The model under review builds one solid part; all positions refer to its coordinate system, in mm. Coordinates: 2 decimals unless noted, no trailing zeros. Write each loop counter-clockwise with the first axis right and the second up, starting at its lowest first coordinate (ties: lowest second). Pieces come first, ordered by that corner, then holes.
```python
from build123d import *

# Parameters (mm, degrees)
SKETCH1_W           = 50
SKETCH1_H           = 14
BOSS_EXTRUDE1_DEPTH = 2.2
SKETCH2_R           = 2.5
CUT_EXTRUDE1_DEPTH  = 27.054558142
FILLET1_R           = 0.1
FILLET2_R           = 0.1


with BuildPart() as part:
    # Sketch1 → Boss-Extrude1 (new body)
    with BuildSketch(Plane(origin=(0, 0, 0), x_dir=(0, 0, -1), z_dir=(1, 0, 0))):
        Rectangle(SKETCH1_W, SKETCH1_H)
    extrude(amount=BOSS_EXTRUDE1_DEPTH)

    # Sketch2 → Cut-Extrude1 (cut, through all)
    with BuildSketch(Plane(origin=(2.2, 0, 0), x_dir=(0, 0, -1), z_dir=(1, 0, 0))):
        with Locations((-20, 0)):
            Circle(SKETCH2_R)
    extrude(amount=-CUT_EXTRUDE1_DEPTH, mode=Mode.SUBTRACT)

    # Fillet1
    fillet1_edges = [part.edges().sort_by_distance(p)[0] for p in [
        (2.2, 0, -25),
    ]]
    fillet(fillet1_edges, radius=FILLET1_R)

    # Fillet2
    fillet2_edges = [part.edges().sort_by_distance(p)[0] for p in [
        (0, 0, -25),
    ]]
    fillet(fillet2_edges, radius=FILLET2_R)


solid = part.part
```
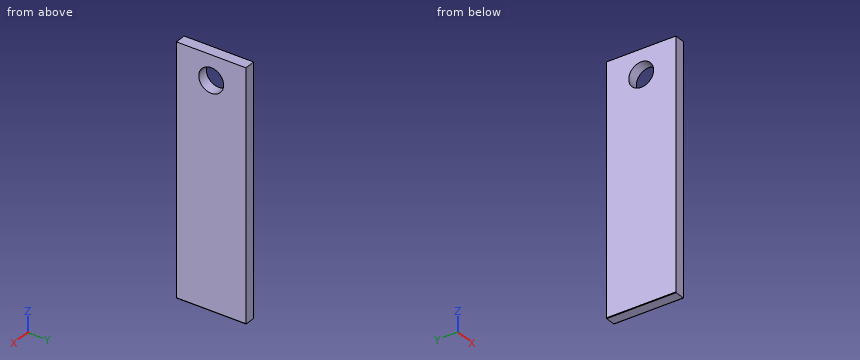
Item 1: To check wall thickness, follow line 1 along Y through (x, z) = (1.5, 20); line 2 along Z through (x, y) = (1.55, 0.25); line 3 along Z through (x, y) = (1.7, 2). State the ranges of each line that lie inside material, in increasing order.
Solved:
line 1: y = -7 to -2.5, 2.5 to 7
line 2: z = -25 to 17.51, 22.49 to 25
line 3: z = -25 to 18.5, 21.5 to 25
Item 2: Take a section at B-B, the plane y = 0. Write out the cut boundary in (x, z).
Solved:
outline: (0, -24.9) arc R0.1 ccw to (0.1, -25) - (2.1, -25) arc R0.1 ccw to (2.2, -24.9) - (2.2, 17.5) - (0, 17.5) - close; (0, 22.5) - (2.2, 22.5) - (2.2, 25) - (0, 25) - close
Item 3: Take a section at A-A, the plane z = 20. Write out the cut boundary in (x, y).
Solved:
outline: (0, -7) - (2.2, -7) - (2.2, -2.5) - (0, -2.5) - close; (0, 2.5) - (2.2, 2.5) - (2.2, 7) - (0, 7) - close
Item 4: Take a section at C-C, the plane x = 1.15. Write out the cut boundary in (y, z), plus the area to 3 significant figures.
Solved:
outline: (-7, -25) - (7, -25) - (7, 25) - (-7, 25) - close; hole circle Ø5 at (0, 20)
area: 680 mm2
